from build123d import *

# Parameters (mm, degrees)
SKETCH1_W            = 38
SKETCH1_H            = 27.444444444
BOSS_EXTRUDE1_DEPTH  = 21
SKETCH2_W            = 8
SKETCH2_H            = 8
BOSS_EXTRUDE2_DEPTH  = 2
SKETCH3_W            = 5.774074058
SKETCH3_H            = 3
CUT_EXTRUDE1_DEPTH   = 2
FILLET1_R            = 2
FILLET2_R            = 1.5
FILLET1_OF_MIRROR1_R = 2
FILLET2_OF_MIRROR1_R = 1.5
SKETCH5_R            = 1.25
BOSS_EXTRUDE3_DEPTH  = 5
SKETCH6_R            = 1.25
BOSS_EXTRUDE4_DEPTH  = 5
FILLET5_R            = 1


with BuildPart() as part:
    # Sketch1 → Boss-Extrude1 (new body)
    with BuildSketch(Plane.XY):
        Rectangle(SKETCH1_W, SKETCH1_H)
    extrude(amount=BOSS_EXTRUDE1_DEPTH)

    # Sketch2 → Boss-Extrude2 (add)
    with BuildSketch(Plane.XY):
        with Locations((-23, 0)):
            Rectangle(SKETCH2_W, SKETCH2_H)
    boss_extrude2 = extrude(amount=BOSS_EXTRUDE2_DEPTH)

    # Sketch3 → Cut-Extrude1 (cut)
    with BuildSketch(Plane.XY.offset(2)):
        with Locations((-24.112962971, 0)):
            Rectangle(SKETCH3_W, SKETCH3_H)
    cut_extrude1 = extrude(amount=-CUT_EXTRUDE1_DEPTH, mode=Mode.SUBTRACT)

    # Fillet1
    fillet1_edges = [part.edges().sort_by_distance(p)[0] for p in [
        (-27, -4, 1),
        (-27, 4, 1),
    ]]
    fillet(fillet1_edges, radius=FILLET1_R)

    # Fillet2
    fillet2_edges = [part.edges().sort_by_distance(p)[0] for p in [
        (-21.225925942, 1.5, 1),
        (-21.225925942, -1.5, 1),
    ]]
    fillet(fillet2_edges, radius=FILLET2_R - 0.0001)  # a hair under: the kernel refuses the full size

    # Mirror1: Boss-Extrude2, Cut-Extrude1 across plane
    add(boss_extrude2.mirror(Plane(origin=(0, 0, 0), x_dir=(0, 0, 1), z_dir=(1, 0, 0))))
    add(cut_extrude1.mirror(Plane(origin=(0, 0, 0), x_dir=(0, 0, 1), z_dir=(1, 0, 0))), mode=Mode.SUBTRACT)

    # Fillet1 of Mirror1
    fillet1_of_mirror1_edges = [part.edges().sort_by_distance(p)[0] for p in [
        (27, -4, 1),
        (27, 4, 1),
    ]]
    fillet(fillet1_of_mirror1_edges, radius=FILLET1_OF_MIRROR1_R)

    # Fillet2 of Mirror1
    fillet2_of_mirror1_edges = [part.edges().sort_by_distance(p)[0] for p in [
        (21.225925942, 1.5, 1),
        (21.225925942, -1.5, 1),
    ]]
    fillet(fillet2_of_mirror1_edges, radius=FILLET2_OF_MIRROR1_R - 0.0001)  # a hair under: the kernel refuses the full size

    # Sketch5 → Boss-Extrude3 (add)
    with BuildSketch(Plane.ZY.offset(19)):
        with Locations(Location((1.25, 10, 0), (0, 0, 180))):
            Circle(SKETCH5_R)
        with Locations(Location((1.25, 6.5, 0), (0, 0, 180))):
            Circle(SKETCH5_R)
    extrude(amount=BOSS_EXTRUDE3_DEPTH)

    # Sketch6 → Boss-Extrude4 (add)
    with BuildSketch(Plane(origin=(19, 0, 0), x_dir=(0, 0, -1), z_dir=(1, 0, 0))):
        with Locations((-1.25, -6.5)):
            Circle(SKETCH6_R)
        with Locations((-1.25, -10)):
            Circle(SKETCH6_R)
    extrude(amount=BOSS_EXTRUDE4_DEPTH)

    # Fillet5
    fillet5_edges = [part.edges().sort_by_distance(p)[0] for p in [
        (19, 13.722222222, 10.5),
        (19, -13.722222222, 10.5),
        (-19, -13.722222222, 10.5),
        (-19, 13.722222222, 10.5),
        (19, 0, 21),
        (0, -13.722222222, 21),
        (-19, 0, 21),
        (0, 13.722222222, 21),
    ]]
    fillet(fillet5_edges, radius=FILLET5_R)


solid = part.part
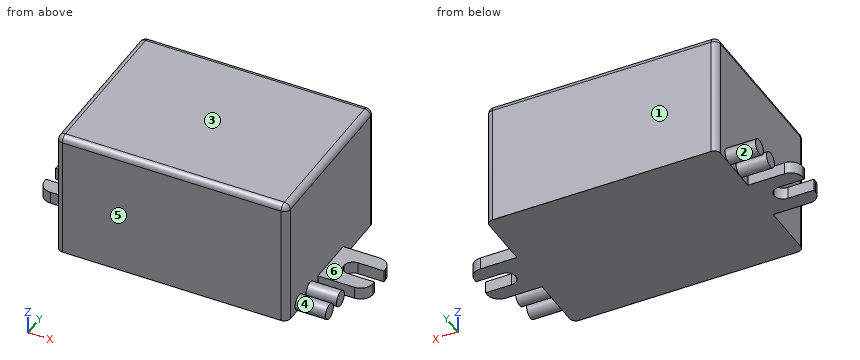
Input: part model. Units: mm. Frame: model coordinates. Face numbers are marked on the shaded views. A direction names the side the tool comes from. Coordinates: 2 decimals unless noted, no trailing zeros. Order: outer loops, then holes, each group sorted by start corner. A loop starts at its lowest first (then second) coordinate and runs counter-clockwise, first axis right, second up. Notation, with made-up numbers: M -24.5,81 L 16.5,81 A8 cw 16.5,90 Z; hole C 12.25,-15.75 d1. An arc over 180 degrees is marked long. Answer as CSV lines item,"result".
1. Material intervals for line 1 (X direction, y = -7, z = 2.5); line 2 (Z direction, x = -21.5, y = -2.25); line 3 (Y direction, x = 18.5, z = 8.5), sorted ascending. Write a range as from..to.
Reported:
line 1,"-19..19"
line 2,"0..2"
line 3,"-13.59..13.59"
2. First-contact query: P1, Ø6, axis at y = -11, z = 12, coming from the +X side; P2, Ø1, axis at x = 23, z = 1, coming from the -Y side; P3, Ø2, axis at x = -24, z = 1.5, coming from the +Y side; P4, Ø1, axis at x = -21, z = 4.5, coming from the -Y side. Flat tips, straight axial feed; report the tip coordinate or a pass-through.
Reported:
P1,"x = 19"
P2,"y = -11.25"
P3,"y = 11.25"
P4,"through"
3. Section A-A (z = 11.25). Return the cut outline in (x, y), then the cut area to 3 significant figures.
Reported:
outline,"M -19,-12.72 A1 ccw -18,-13.72 L 18,-13.72 A1 ccw 19,-12.72 L 19,12.72 A1 ccw 18,13.72 L -18,13.72 A1 ccw -19,12.72 Z"
area,"1,040 mm2"
4. Access query for the marked faces 4, 5 and 6. Directions: +Z, -Z, +X, -X, +Y, -Y. A direction counts if a zero-diameter tool reaches every point of the face in a straight line with its end or side. Return the directions, or none.
Reported:
face 4,"+X"
face 5,"+Z, -Z, +X, -X, -Y"
face 6,"+Z, +X, +Y"
5. Pull-direction query (Y, two-part tool) for the marked faces 1, 2 and 3; classes: released by +Y, released by -Y, zero draft, split by the parting line, or undercut.
Reported:
face 1,"released by +Y"
face 2,"undercut"
face 3,"zero draft"
